The listing builds one solid part. Answer for the finished solid, in the listing's coordinates (mm). Face numbers are marked on the shaded views. A direction names the side the tool comes from. Round coordinates to 2 decimals unless told otherwise and drop trailing zeros. Loops run counter-clockwise (first coordinate to the right, second up) from the corner with the lowest first, then second, coordinate; pieces in that order, holes last. Notation, with made-up numbers: (-11.5, 49.25) - (17.5, 49.25) arc R17 cw to (17.5, 78.25) - close; hole circle Ø9 at (49, -27.5). An arc over 180 degrees is marked (long way). One line per item, written item: value.
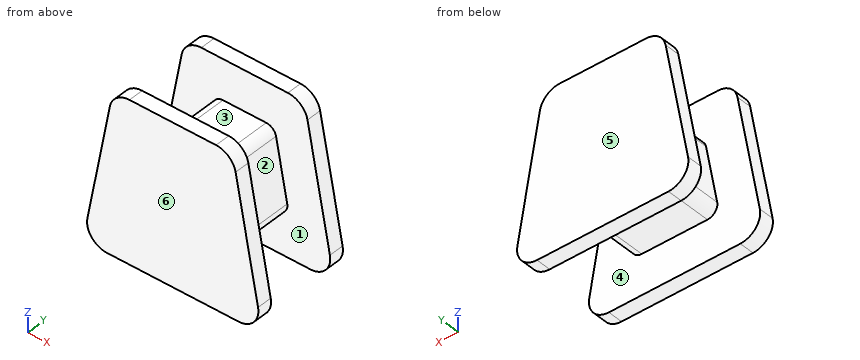
```python
from build123d import *

# Parameters (mm, degrees)
BOSS_EXTRUDE1_DEPTH = 12.7
CUT_EXTRUDE1_DEPTH  = 8.89


with BuildPart() as part:
    # Sketch1 → Boss-Extrude1 (new, symmetric)
    with BuildSketch(Plane(origin=(0, 0, 0), x_dir=(1, 0, 0), z_dir=(0, 1, 0))):
        with BuildLine():
            Line((-16.738974461, 20.32), (16.738974461, 20.32))
            ThreePointArc((16.738974461, 20.32), (20.64808073, 18.484270053), (21.73196517, 14.303814242))
            Line((21.73196517, 14.303814242), (16.01696517, -16.176185758))
            ThreePointArc((16.01696517, -16.176185758), (14.268244513, -19.149106269), (11.023974461, -20.32))
            Line((11.023974461, -20.32), (-11.023974461, -20.32))
            ThreePointArc((-11.023974461, -20.32), (-14.268244513, -19.149106269), (-16.01696517, -16.176185758))
            Line((-16.01696517, -16.176185758), (-21.73196517, 14.303814242))
            ThreePointArc((-21.73196517, 14.303814242), (-20.64808073, 18.484270053), (-16.738974461, 20.32))
        make_face()
    extrude(amount=BOSS_EXTRUDE1_DEPTH, both=True)

    # Sketch3 → Cut-Extrude1 (cut, symmetric)
    with BuildSketch(Plane(origin=(0, 0, 0), x_dir=(1, 0, 0), z_dir=(0, 1, 0))):
        with BuildLine():
            Line((-16.738974461, 20.32), (16.738974461, 20.32))
            ThreePointArc((16.738974461, 20.32), (20.64808073, 18.484270053), (21.73196517, 14.303814242))
            Line((21.73196517, 14.303814242), (16.01696517, -16.176185758))
            ThreePointArc((16.01696517, -16.176185758), (14.268244513, -19.149106269), (11.023974461, -20.32))
            Line((11.023974461, -20.32), (-11.023974461, -20.32))
            ThreePointArc((-11.023974461, -20.32), (-14.268244513, -19.149106269), (-16.01696517, -16.176185758))
            Line((-16.01696517, -16.176185758), (-21.73196517, 14.303814242))
            ThreePointArc((-21.73196517, 14.303814242), (-20.64808073, 18.484270053), (-16.738974461, 20.32))
        make_face()
        with BuildLine():
            Line((5.51198723, -10.16), (-5.51198723, -10.16))
            ThreePointArc((-5.51198723, -10.16), (-7.134122257, -9.574553135), (-8.008482585, -8.088092879))
            Line((-8.008482585, -8.088092879), (-10.865982585, 7.151907121))
            ThreePointArc((-10.865982585, 7.151907121), (-10.324040365, 9.242135026), (-8.36948723, 10.16))
            Line((-8.36948723, 10.16), (8.36948723, 10.16))
            ThreePointArc((8.36948723, 10.16), (10.324040365, 9.242135026), (10.865982585, 7.151907121))
            Line((10.865982585, 7.151907121), (8.008482585, -8.088092879))
            ThreePointArc((8.008482585, -8.088092879), (7.134122257, -9.574553135), (5.51198723, -10.16))
        make_face(mode=Mode.SUBTRACT)
    extrude(amount=CUT_EXTRUDE1_DEPTH, both=True, mode=Mode.SUBTRACT)


solid = part.part
```
1) A cutting plane is placed at C-C on x = -18. Give the vertices of the cut face in (y, z).
Final values:
outline: (-12.7, -20.16) - (-8.89, -20.16) - (-8.89, 5.6) - (-12.7, 5.6) - close; (8.89, -20.16) - (12.7, -20.16) - (12.7, 5.6) - (8.89, 5.6) - close
2) A cutting plane is placed at D-D on y = 0. Give the vertices of the cut face in (x, z).
Final values:
outline: (-10.87, -7.15) arc R2.54 ccw to (-8.37, -10.16) - (8.37, -10.16) arc R2.54 ccw to (10.87, -7.15) - (8.01, 8.09) arc R2.54 ccw to (5.51, 10.16) - (-5.51, 10.16) arc R2.54 ccw to (-8.01, 8.09) - close
3) For the marked faces 1, 2 and 3, determine the directions among +Z, -Z, +X, -X, +Y, -Y from which every point of the face is accessible in a straight line to the end or side of a thin tool.
Final values:
face 1: none
face 2: +Z, +X
face 3: +Z, +X, -X
4) For a pull along Y with two mould halves and no side action, classify the marked faces 4, 5 and 6 as released by +Y, released by -Y, zero draft, split by the parting line, or undercut.
Final values:
face 4: undercut
face 5: released by +Y
face 6: released by -Y
5) Each of these flat-tipped pins is pushed along its axis until it touches: pin 1 Ø1 at (y, z) = (-8.5, 11.5) entering from -X; pin 2 Ø3 at (x, y) = (5, -0.5) entering from +Z; pin 3 Ø8.5 at (x, y) = (-3, 3.5) entering from -Z. Where does it stop, or does it pass through?
Final values:
pin 1: x = -16.95
pin 2: z = 10.16
pin 3: z = -10.16
6) A cutting plane is placed at B-B on x = 1.5. Give the vertices of the cut face in (y, z), and give its area (3 significant figures).
Final values:
outline: (-12.7, -20.32) - (-8.89, -20.32) - (-8.89, -10.16) - (8.89, -10.16) - (8.89, -20.32) - (12.7, -20.32) - (12.7, 20.32) - (8.89, 20.32) - (8.89, 10.16) - (-8.89, 10.16) - (-8.89, 20.32) - (-12.7, 20.32) - close
area: 671 mm2
7) Consider L1, parallel to Y at x = 7.5, z = 17; L2, parallel to Z at x = -1.5, y = -3.75; L3, parallel to X at y = 2.25, z = -7.5. Determine where each line is inside the solid, lowest interval first.
Final values:
L1: -12.7 to -8.89, 8.89 to 12.7
L2: -10.16 to 10.16
L3: -10.91 to 10.91
8) A cutting plane is placed at A-A on z = 12. Give the vertices of the cut face in (x, y), and give its area (3 significant figures).
Final values:
outline: (-16.8, -12.7) - (16.8, -12.7) - (16.8, -8.89) - (-16.8, -8.89) - close; (-16.8, 8.89) - (16.8, 8.89) - (16.8, 12.7) - (-16.8, 12.7) - close
area: 256 mm2
